Could you check a few things on this model? Use its own coordinates, in mm. A direction names the side the tool comes from. Coordinates: 2 decimals unless noted, no trailing zeros. Loops run counter-clockwise (first coordinate to the right, second up) from the corner with the lowest first, then second, coordinate; pieces in that order, holes last. Notation, with made-up numbers: (33.25, 47) - (62.25, 47) arc R19 cw to (62.25, 56) - close; hole circle Ø1 at (23.25, 26.25). An arc over 180 degrees is marked (long way). One line per item, written item: value. Start each with the question number.
(1) If I drill on line 1 along X through (y, z) = (11, 27); line 2 along Y through (x, z) = (-18.1, 101.6); line 3 along Z through (x, y) = (-18, 30), over which ranges is the centre line in solid material (lowest first)? Write a range as from..to.
(2) On a 3-axis mill with a long thin cutter (end or side, diameter ignored), from which of +Z, -Z, +X, -X, +Y, -Y can I reach the whole of each face in a straight line? I mean faces 5 (the face through (16.806, 28.155, 13.383)), 6 (the face through (-1, 3.175, 95)), 7 (the face through (-1, 2, 76.2)). Say none if no direction works.
(3) I'm going to push a flat-ended pin straight in: P1, Ø1.6, axis at x = -4, y = 2.5, coming from the -Z side. Where does the tip first touch, or does it pass through?
(4) If we section it at A-A on y = 30.48: Write out the boundary of the cut face in (x, z).
(5) If we mould it in two halves opening along X, with no side actions, what happens to faces 1 (the face through (-18.12, 29.57, 99.4)), 2 (the face through (-19.729, 19, 56)), 3 (the face through (-1, 2, 68.262)), 4 (the face through (-0.59, 2.206, 1.003))? For each: pulls with the +X half, pulls with the -X half, needs draft (parallel to the pull), parting line crosses it, or undercut.
(6) If we section it at B-B on z = 101.6: Write out the boundary of the cut face in (x, y) (3 decimals).
(7) If we section it at D-D on y = 35: Write out the boundary of the cut face in (x, z).
(8) If we section it at C-C on x = 9.5: Write out the boundary of the cut face in (y, z) (1 decimal).
```python
from build123d import *

# Parameters (mm, degrees)
BOSS_EXTRUDE1_DEPTH = 114.3
CUT_EXTRUDE1_DEPTH  = 98.425
SKETCH3_R           = 2.38125
CUT_EXTRUDE2_DEPTH  = 98.425
SKETCH4_W           = 31.75
SKETCH4_H           = 7.9375
CUT_EXTRUDE4_DEPTH  = 122.134097336


with BuildPart() as part:
    # Sketch1 → Boss-Extrude1 (new body)
    with BuildSketch(Plane.XY):
        Polygon((18.371241491, 0), (-19.728758509, 0), (-19.728758509, 38.1), (-16.553758509, 38.1), (-16.553758509, 3.175), (15.196241491, 3.175), (15.196241491, 38.1), (18.371241491, 38.1), align=None)
    extrude(amount=BOSS_EXTRUDE1_DEPTH)

    # Sketch2 → Cut-Extrude1 (cut)
    with BuildSketch(Plane(origin=(0, 38.1, 0), x_dir=(1, 0, 0), z_dir=(0, 1, 0))):
        Polygon((-19.728758509, 0), (18.371241491, 0), (18.371241491, -1.996736391), align=None)
    extrude(amount=-CUT_EXTRUDE1_DEPTH, mode=Mode.SUBTRACT)

    # Sketch3 → Cut-Extrude2 (cut)
    with BuildSketch(Plane(origin=(18.371241491, 0, 0), x_dir=(0, 0, -1), z_dir=(1, 0, 0))):
        with Locations((-12.866394699, 30.48)):
            Circle(SKETCH3_R)
        with Locations((-101.6, 30.48)):
            Circle(SKETCH3_R)
    extrude(amount=-CUT_EXTRUDE2_DEPTH, mode=Mode.SUBTRACT)

    # Sketch4 → Cut-Extrude4 (cut, through all)
    with BuildSketch(Plane(origin=(0, 3.175, 0), x_dir=(1, 0, 0), z_dir=(0, 1, 0))):
        with Locations((-0.678758509, -72.23125)):
            Rectangle(SKETCH4_W, SKETCH4_H)
    extrude(amount=-CUT_EXTRUDE4_DEPTH, mode=Mode.SUBTRACT)


solid = part.part
```
Values:
1. line 1: x = -19.73..-16.55, 15.2..18.37
1. line 2: y = 0..28.1, 32.86..38.1
1. line 3: z = 0.09..10.53, 15.2..99.27, 103.93..114.3
2. face 5: +X, -X
2. face 6: +Z, -Z, +Y
2. face 7: +Y, -Y
3. P1: stops at z = 0.78
4. outline: (-19.73, 0) - (-16.55, 0.17) - (-16.55, 10.49) - (-19.73, 10.49) - close; (-19.73, 15.25) - (-16.55, 15.25) - (-16.55, 99.22) - (-19.73, 99.22) - close; (-19.73, 103.98) - (-16.55, 103.98) - (-16.55, 114.3) - (-19.73, 114.3) - close; (15.2, 1.83) - (18.37, 2) - (18.37, 10.49) - (15.2, 10.49) - close; (15.2, 15.25) - (18.37, 15.25) - (18.37, 99.22) - (15.2, 99.22) - close; (15.2, 103.98) - (18.37, 103.98) - (18.37, 114.3) - (15.2, 114.3) - close
5. face 1: needs draft
5. face 2: pulls with the -X half
5. face 3: undercut
5. face 4: pulls with the +X half
6. outline: (-19.729, 0) - (18.371, 0) - (18.371, 28.099) - (15.196, 28.099) - (15.196, 3.175) - (-16.554, 3.175) - (-16.554, 28.099) - (-19.729, 28.099) - close; (-19.729, 32.861) - (-16.554, 32.861) - (-16.554, 38.1) - (-19.729, 38.1) - close; (15.196, 32.861) - (18.371, 32.861) - (18.371, 38.1) - (15.196, 38.1) - close
7. outline: (-19.73, 0) - (-16.55, 0.17) - (-16.55, 114.3) - (-19.73, 114.3) - close; (15.2, 1.83) - (18.37, 2) - (18.37, 114.3) - (15.2, 114.3) - close
8. outline: (0, 1.5) - (3.2, 1.5) - (3.2, 68.3) - (0, 68.3) - close; (0, 76.2) - (3.2, 76.2) - (3.2, 114.3) - (0, 114.3) - close
